from build123d import *

# Parameters (mm, degrees)
EXTRUDE_1_DEPTH     = 16
SKETCH_2_R          = 19
EXTRUDE_2_DEPTH     = 2
SKETCH_3_R          = 19
EXTRUDE_3_DEPTH     = 2
SKETCH_4_R          = 9
SKETCH_4_R_2        = 3.1
EXTRUDE_4_DEPTH     = 8
SKETCH_5_R          = 2
CUT_EXTRUDE_1_DEPTH = 20


with BuildPart() as part:
    # Эскиз1 → Бобышка-Вытянуть1 (new body)
    with BuildSketch(Plane.XY):
        with BuildLine():
            ThreePointArc((-1.498740073, 18.241032987), (-2.492190095, 18.132029527), (-3.478209077, 17.968961235))
            ThreePointArc((-3.478209077, 17.968961235), (-4.533260247, 16.179417721), (-6.364534528, 17.16025077))
            ThreePointArc((-6.364534528, 17.16025077), (-7.291735947, 16.787259846), (-8.197195372, 16.364213831))
            ThreePointArc((-8.197195372, 16.364213831), (-8.73030932, 14.356382045), (-10.758300573, 14.806771256))
            ThreePointArc((-10.758300573, 14.806771256), (-11.550487101, 14.197455898), (-12.308233185, 13.545807547))
            ThreePointArc((-12.308233185, 13.545807547), (-12.27987129, 11.468599189), (-14.35417268, 11.355141255))
            ThreePointArc((-14.35417268, 11.355141255), (-14.952591467, 10.554691596), (-15.50642565, 9.722770687))
            ThreePointArc((-15.50642565, 9.722770687), (-14.918691382, 7.730242796), (-16.885461466, 7.061352373))
            ThreePointArc((-16.885461466, 7.061352373), (-17.245730527, 6.129134102), (-17.554577461, 5.178640403))
            ThreePointArc((-17.554577461, 5.178640403), (-16.451060383, 3.418569659), (-18.164432821, 2.243855289))
            ThreePointArc((-18.164432821, 2.243855289), (-18.259832648, 1.249006771), (-18.300786569, 0.250434051))
            ThreePointArc((-18.300786569, 0.250434051), (-16.763329494, -1.146643151), (-18.09623129, -2.740058277))
            ThreePointArc((-18.09623129, -2.740058277), (-17.919686515, -3.723753679), (-17.689710057, -4.696345849))
            ThreePointArc((-17.689710057, -4.696345849), (-15.832339144, -5.626814684), (-16.685915069, -7.520754256))
            ThreePointArc((-16.685915069, -7.520754256), (-16.25051921, -8.420340353), (-15.766668676, -9.294819262))
            ThreePointArc((-15.766668676, -9.294819262), (-13.727136627, -9.689671112), (-14.03808086, -11.743670296))
            ThreePointArc((-14.03808086, -11.743670296), (-13.376125236, -12.492428904), (-12.674285607, -13.203938451))
            ThreePointArc((-12.674285607, -13.203938451), (-10.603855185, -13.033888962), (-10.349106414, -15.095612034))
            ThreePointArc((-10.349106414, -15.095612034), (-9.509685246, -15.638011152), (-8.641908755, -16.133781929))
            ThreePointArc((-8.641908755, -16.133781929), (-6.694134312, -15.411442894), (-5.892586089, -17.327981286))
            ThreePointArc((-5.892586089, -17.327981286), (-4.937955404, -17.623793652), (-3.968601065, -17.867056608))
            ThreePointArc((-3.968601065, -17.867056608), (-2.287940121, -16.646000608), (-0.999039611, -18.275213435))
            ThreePointArc((-0.999039611, -18.275213435), (0, -18.3025), (0.999039611, -18.275213435))
            ThreePointArc((0.999039611, -18.275213435), (2.287940121, -16.646000608), (3.968601065, -17.867056608))
            ThreePointArc((3.968601065, -17.867056608), (4.937955404, -17.623793652), (5.892586089, -17.327981286))
            ThreePointArc((5.892586089, -17.327981286), (6.694134312, -15.411442894), (8.641908755, -16.133781929))
            ThreePointArc((8.641908755, -16.133781929), (9.509685246, -15.638011152), (10.349106414, -15.095612034))
            ThreePointArc((10.349106414, -15.095612034), (10.603855185, -13.033888962), (12.674285607, -13.203938451))
            ThreePointArc((12.674285607, -13.203938451), (13.376125236, -12.492428904), (14.03808086, -11.743670296))
            ThreePointArc((14.03808086, -11.743670296), (13.727136627, -9.689671112), (15.766668676, -9.294819262))
            ThreePointArc((15.766668676, -9.294819262), (16.25051921, -8.420340353), (16.685915069, -7.520754256))
            ThreePointArc((16.685915069, -7.520754256), (15.832339144, -5.626814684), (17.689710057, -4.696345849))
            ThreePointArc((17.689710057, -4.696345849), (17.919686515, -3.723753679), (18.09623129, -2.740058277))
            ThreePointArc((18.09623129, -2.740058277), (16.763329494, -1.146643151), (18.300786569, 0.250434051))
            ThreePointArc((18.300786569, 0.250434051), (18.259832648, 1.249006771), (18.164432821, 2.243855289))
            ThreePointArc((18.164432821, 2.243855289), (16.451060383, 3.418569659), (17.554577461, 5.178640403))
            ThreePointArc((17.554577461, 5.178640403), (17.245730527, 6.129134102), (16.885461466, 7.061352373))
            ThreePointArc((16.885461466, 7.061352373), (14.918691382, 7.730242796), (15.50642565, 9.722770687))
            ThreePointArc((15.50642565, 9.722770687), (14.952591467, 10.554691596), (14.35417268, 11.355141255))
            ThreePointArc((14.35417268, 11.355141255), (12.27987129, 11.468599189), (12.308233185, 13.545807547))
            ThreePointArc((12.308233185, 13.545807547), (11.550487101, 14.197455898), (10.758300573, 14.806771256))
            ThreePointArc((10.758300573, 14.806771256), (8.73030932, 14.356382045), (8.197195372, 16.364213831))
            ThreePointArc((8.197195372, 16.364213831), (7.291735947, 16.787259846), (6.364534528, 17.16025077))
            ThreePointArc((6.364534528, 17.16025077), (4.533260247, 16.179417721), (3.478209077, 17.968961235))
            ThreePointArc((3.478209077, 17.968961235), (2.492190095, 18.132029527), (1.498740073, 18.241032987))
            ThreePointArc((1.498740073, 18.241032987), (0, 16.8025), (-1.498740073, 18.241032987))
        make_face()
    extrude(amount=EXTRUDE_1_DEPTH)

    # Эскиз2 → Бобышка-Вытянуть2 (add)
    with BuildSketch(Plane(origin=(0, 0, 0), x_dir=(-1, 0, 0), z_dir=(0, 0, -1))):
        Circle(SKETCH_2_R)
    extrude(amount=EXTRUDE_2_DEPTH)

    # Эскиз3 → Бобышка-Вытянуть3 (add)
    with BuildSketch(Plane.XY.offset(16)):
        Circle(SKETCH_3_R)
    extrude(amount=EXTRUDE_3_DEPTH)

    # Эскиз4 → Бобышка-Вытянуть4 (add)
    with BuildSketch(Plane.XY.offset(18)):
        Circle(SKETCH_4_R)
        Circle(SKETCH_4_R_2, mode=Mode.SUBTRACT)
    extrude(amount=EXTRUDE_4_DEPTH)

    # Эскиз5 → Вырез-Вытянуть1 (cut, through all)
    with BuildSketch(Plane(origin=(0, 0, 0), x_dir=(0, 0, -1), z_dir=(1, 0, 0))):
        with Locations((-22.5, 0)):
            Circle(SKETCH_5_R)
    extrude(amount=-CUT_EXTRUDE_1_DEPTH, mode=Mode.SUBTRACT)


solid = part.part
Source: CAD feature listing. Evaluate the final solid. Frame: model axes, mm. A direction names the side the tool comes from. Coordinates: 2 decimals unless noted, no trailing zeros. Loops run counter-clockwise (first coordinate to the right, second up) from the corner with the lowest first, then second, coordinate; pieces in that order, holes last. Notation, with made-up numbers: (46.5, 8.5) - (82.5, 8.5) arc R16 cw to (82.5, 15.5) - close; hole circle Ø3 at (75.5, 5.5). An arc over 180 degrees is marked (long way). One line per item, written item: value. Start each with the question number.
1. Set-up query: faces 4 (the cylindrical face through (-7.279, 16.793, 7.888)), 5 (the cylindrical face through (-17.923, -3.71, 7.888)), 6 (the cylindrical face through (10.579, -13.054, 7.888)). Return all of +Z, -Z, +X, -X, +Y, -Y with unobstructed straight access to the full face (end or side cutting, diameter ignored); none if empty.
2. Section C-C (z = 22.5). Return the cut outline in (x, y).
3. Ray query, L1, parallel to Z at x = 4, y = 17.5; L2, parallel to X at y = -17, z = 12; L3, parallel to Z at x = 1, y = 12.5. Return the intervals inside material, ascending.
4. Section B-B (y = -5.5). Return the cut outline in (x, z).
5. Section A-A (x = 0). Return the cut outline in (y, z), and give its area (3 significant figures).
6. Contact query for flat-ended pins moving along their axis: P1, Ø10, axis at x = 11, y = -10.5, coming from the +Z side; P2, Ø3, axis at y = -3, z = 16.5, coming from the -X side; P3, Ø5, axis at x = 2, z = 6, coming from the +Y side. Output: stop coordinate, or through.
7. Mould query, pull axis Z, two halves, no side actions, for faces 1 (the flat face through (0, 0, -2)), 2 (the flat face through (0, 0, 18)), 3 (the cylindrical face through (-13.39, -12.48, 7.89)). Classes: pulls with the +Z half, pulls with the -Z half, needs draft (parallel to the pull), parting line crosses it, or undercut.
8. Section D-D (y = 13). Return the cut outline in (x, z).
Verdict:
1. face 4: -X, +Y
1. face 5: -X, -Y
1. face 6: none
2. outline: (-8.77, -2) arc R9 ccw (long way) to (-8.77, 2) - (-2.37, 2) arc R3.1 cw (long way) to (-2.37, -2) - close
3. L1: z = -2 to 0, 16 to 18
3. L2: x = -5.81 to -3.48, -1.51 to 1.51, 3.48 to 5.81
3. L3: z = -2 to 18
4. outline: (-18.19, -2) - (18.19, -2) - (18.19, 0) - (15.88, 0) - (15.88, 16) - (18.19, 16) - (18.19, 18) - (7.12, 18) - (7.12, 26) - (-7.12, 26) - (-7.12, 18) - (-18.19, 18) - (-18.19, 16) - (-15.88, 16) - (-15.88, 0) - (-18.19, 0) - close
5. outline: (-19, -2) - (19, -2) - (19, 0) - (16.8, 0) - (16.8, 16) - (19, 16) - (19, 18) - (9, 18) - (9, 26) - (3.1, 26) - (3.1, 18) - (-3.1, 18) - (-3.1, 26) - (-9, 26) - (-9, 18) - (-19, 18) - (-19, 16) - (-18.3, 16) - (-18.3, 0) - (-19, 0) - close
5. area: 808 mm2
6. P1: stops at z = 18
6. P2: stops at x = -18.94
6. P3: stops at y = 18.24
7. face 1: pulls with the -Z half
7. face 2: pulls with the +Z half
7. face 3: undercut
8. outline: (-13.86, -2) - (13.86, -2) - (13.86, 0) - (11.96, 0) - (11.96, 16) - (13.86, 16) - (13.86, 18) - (-13.86, 18) - (-13.86, 16) - (-11.96, 16) - (-11.96, 0) - (-13.86, 0) - close
